For this review, take the finished solid that the model builds, in its own axes (mm). A direction names the side the tool comes from. Give positions to 0.01 mm unless a question says otherwise; leave off trailing zeros. Write each loop counter-clockwise with the first axis right and the second up, starting at its lowest first coordinate (ties: lowest second). Pieces come first, ordered by that corner, then holes.
Q1. Machinability: for faces 5 (the flat face through (15, 13, -3)), 6 (the flat face through (11, 11, 61.932)), 7 (the flat face through (19, 12, -3)), which of the approach directions +Z, -Z, +X, -X, +Y, -Y give a long, thin tool a straight path to every point of the face, cutting with its end or side? Answer none if there is none.
Q2. We need section C-C (z = 60.5). Write out the cut boundary in (x, y).
Q3. For line 1 (Y direction, x = 10.5, z = 36); line 2 (Y direction, x = 9.5, z = 60); line 3 (Z direction, x = 9.75, y = 11.75), list the stretches that pass through material, from the lowest coordinate up.
Q4. We need section B-B (x = 5.25). Write out the cut boundary in (y, z), then the cut area to 3 significant figures.
Q5. We need section A-A (z = 33). Write out the cut boundary in (x, y), then the cut area to 3 significant figures.
Q6. Insertion check: P1, Ø5, axis at x = 7, y = 10.5, coming from the +Z side; P2, Ø2, axis at x = 9.5, z = 3.5, coming from the -Y side; P3, Ø1, axis at x = 13, y = 5.5, coming from the -Z side; P4, Ø5, axis at x = 17.5, z = 67, coming from the -Y side. Each pin has a flat end and moves straight along its axis. Give the tip position at first contact, or say it passes through.
Q7. Mouldability with a two-part tool opening along Z and no side actions: class faces 1 (the flat face through (11, 8, 0)), 2 (the cylindrical face through (11.154, 0.782, 54.735)), 3 (the flat face through (11, 9.6, 3)), 4 (the flat face through (11, 0, 25)) as released by +Z, released by -Z, zero draft, split by the parting line, or undercut.
```python
from build123d import *

# Parameters (mm, degrees)
SKETCH_1_W      = 22
SKETCH_1_H      = 15
EXTRUDE_1_DEPTH = 2
SKETCH_2_W      = 22
SKETCH_2_H      = 30
EXTRUDE_2_DEPTH = 2
EXTRUDE_3_DEPTH = 22
SKETCH_4_W      = 8
SKETCH_4_H      = 3
EXTRUDE_4_DEPTH = 6
SKETCH_5_W      = 8
SKETCH_5_H      = 3
EXTRUDE_5_DEPTH = 6
CHAMFER_1_SIZE  = 2
SKETCH_6_W      = 2
SKETCH_6_H      = 1
EXTRUDE_6_DEPTH = 22
FILLET_1_R      = 10


with BuildPart() as part:
    # 草图1 → 凸台-拉伸1 (new body)
    with BuildSketch(Plane.XY):
        with Locations((11, 7.5)):
            Rectangle(SKETCH_1_W, SKETCH_1_H)
    extrude(amount=EXTRUDE_1_DEPTH)

    # 草图2 → 凸台-拉伸2 (add)
    with BuildSketch(Plane.XZ):
        with Locations((11, 15)):
            Rectangle(SKETCH_2_W, SKETCH_2_H)
    extrude(amount=-EXTRUDE_2_DEPTH)

    # 草图3 → 凸台-拉伸3 (add)
    with BuildSketch(Plane.ZY):
        Polygon((64, 15), (0, 15), (0, 13), (61.931971091, 13), (61.931971091, 10.452580583), (61.931971091, 9.760398216), (60.906850806, 8.735277931), (55.196693161, 3.025120286), (54.171572875, 2), (53.479390508, 2), (30, 2), (30, 0), (55, 0), (64, 9), align=None)
    extrude(amount=-EXTRUDE_3_DEPTH)

    # 草图4 → 凸台-拉伸4 (add)
    with BuildSketch(Plane.XY.offset(64)):
        with Locations((18, 13.5)):
            Rectangle(SKETCH_4_W, SKETCH_4_H)
    extrude(amount=EXTRUDE_4_DEPTH)

    # 草图5 → 凸台-拉伸5 (add)
    with BuildSketch(Plane(origin=(0, 0, 0), x_dir=(-1, 0, 0), z_dir=(0, 0, -1))):
        with Locations((-18, 13.5)):
            Rectangle(SKETCH_5_W, SKETCH_5_H)
    extrude(amount=EXTRUDE_5_DEPTH)

    # 倒角1
    chamfer_1_edges = [part.edges().sort_by_distance(p)[0] for p in [
        (14, 12, 67),
        (14, 12, -3),
    ]]
    chamfer(chamfer_1_edges, length=CHAMFER_1_SIZE)

    # 草图6 → 凸台-拉伸6 (add)
    with BuildSketch(Plane.ZY):
        Polygon((57.171572875, 7), (59.171572875, 7), (59.171572875, 8.6), (57.171572875, 8.6), (57.171572875, 9.6), (61.771572875, 9.6), (61.771572875, 7.925359102), (60.513582407, 7.925359102), (60.513582407, 6.316484683), (59.171572875, 6.316484683), (59.171572875, 5), (57.171572875, 5), align=None)
        with Locations((3, 6.5)):
            Rectangle(SKETCH_6_W, SKETCH_6_H)
        with Locations((3, 9.1)):
            Rectangle(SKETCH_6_W, SKETCH_6_H)
    extrude(amount=-EXTRUDE_6_DEPTH)

    # 圆角1
    fillet_1_edges = [part.edges().sort_by_distance(p)[0] for p in [
        (11, 2, 54.171572875),
        (11, 0, 55),
    ]]
    fillet(fillet_1_edges, radius=FILLET_1_R)


solid = part.part
```
Computed:
1. face 5: -Z, -X, -Y
1. face 6: +X, -X
1. face 7: -Z, +X, -X, -Y
2. outline: (0, 5.5) - (22, 5.5) - (22, 9.6) - (0, 9.6) - close; (0, 13) - (22, 13) - (22, 15) - (0, 15) - close
3. line 1: y = 0 to 2, 13 to 15
3. line 2: y = 5 to 9.6, 13 to 15
3. line 3: z = 0 to 2, 61.93 to 64
4. outline: (0, 0) - (15, 0) - (15, 64) - (9, 64) - (2.93, 57.93) arc R10 ccw to (0, 50.86) - close; hole (2, 2) - (6, 2) - (6, 4) - (7, 4) - (7, 2) - (8.6, 2) - (8.6, 4) - (9.6, 4) - (9.6, 2) - (13, 2) - (13, 61.93) - (9.76, 61.93) - (9.6, 61.77) - (9.6, 57.17) - (8.6, 57.17) - (8.6, 59.17) - (7, 59.17) - (7, 57.17) - (5, 57.17) - (4.93, 57.1) arc R10 ccw to (2, 50.03) - close
4. area: 302 mm2
5. outline: (0, 0) - (22, 0) - (22, 2) - (0, 2) - close; (0, 13) - (22, 13) - (22, 15) - (0, 15) - close
5. area: 88.0 mm2
6. P1: stops at z = 64
6. P2: stops at y = 0
6. P3: stops at z = 0
6. P4: stops at y = 12
7. face 1: released by -Z
7. face 2: released by +Z
7. face 3: undercut
7. face 4: zero draft
